from build123d import *

# Parameters (mm, degrees)
SKETCH1_W                  = 109.5
SKETCH1_H                  = 83
BOSS_EXTRUDE1_DEPTH        = 2
F_3_2_3_2_DIAMETER_HOLE2_D = 3.2
F_2_6_2_6_DIAMETER_HOLE2_D = 2.6
F_2_6_2_6_DIAMETER_HOLE1_D = 2.6
SKETCH9_R                  = 3
CUT_EXTRUDE1_DEPTH         = 1
F_2_2_2_2_DIAMETER_HOLE1_D = 2.2
FILLET1_R                  = 1
FILLET2_R                  = 3


with BuildPart() as part:
    # Sketch1 → Boss-Extrude1 (new body)
    with BuildSketch(Plane.XY):
        with Locations((0, -41.5)):
            Rectangle(SKETCH1_W, SKETCH1_H)
        with BuildLine():
            Line((-44.75, -31.5), (-48.75, -31.5))
            Line((-48.75, -31.5), (-48.75, -51.5))
            Line((-48.75, -51.5), (-44.75, -51.5))
            Line((-44.75, -51.5), (-44.75, -74))
            ThreePointArc((-44.75, -74), (-43.871320344, -76.121320344), (-41.75, -77))
            Line((-41.75, -77), (41.75, -77))
            ThreePointArc((41.75, -77), (43.871320344, -76.121320344), (44.75, -74))
            Line((44.75, -74), (44.75, -51.5))
            Line((44.75, -51.5), (48.75, -51.5))
            Line((48.75, -51.5), (48.75, -41.5))
            Line((48.75, -41.5), (48.75, -31.5))
            Line((48.75, -31.5), (44.75, -31.5))
            Line((44.75, -31.5), (44.75, -19.1))
            ThreePointArc((44.75, -19.1), (43.871320344, -16.978679656), (41.75, -16.1))
            Line((41.75, -16.1), (31.75, -16.1))
            ThreePointArc((31.75, -16.1), (29.628679656, -15.221320344), (28.75, -13.1))
            Line((28.75, -13.1), (28.75, -9))
            ThreePointArc((28.75, -9), (27.871320344, -6.878679656), (25.75, -6))
            Line((25.75, -6), (-41.75, -6))
            ThreePointArc((-41.75, -6), (-43.871320344, -6.878679656), (-44.75, -9))
            Line((-44.75, -9), (-44.75, -31.5))
        make_face(mode=Mode.SUBTRACT)
    extrude(amount=BOSS_EXTRUDE1_DEPTH)

    # Ø3.2 (3.2) Diameter Hole2 (through all)
    with Locations(Plane.XY.offset(2)):
        with Locations((-48.25, -3.5), (-48.25, -79.5), (48.25, -79.5), (48.25, -3.5)):
            Hole(F_3_2_3_2_DIAMETER_HOLE2_D / 2)

    # Ø2.6 (2.6) Diameter Hole2 (through all)
    with Locations(Plane.XY.offset(2)):
        with Locations((33.65, -11.6)):
            Hole(F_2_6_2_6_DIAMETER_HOLE2_D / 2)

    # Ø2.6 (2.6) Diameter Hole1 (through all)
    with Locations(Plane.XY.offset(2)):
        with Locations((33.65, -2.07)):
            Hole(F_2_6_2_6_DIAMETER_HOLE1_D / 2)

    # Sketch9 → Cut-Extrude1 (cut)
    with BuildSketch(Plane.XY.offset(2)):
        with Locations((-48.25, -3.5)):
            Circle(SKETCH9_R)
        with Locations((48.25, -3.5)):
            Circle(SKETCH9_R)
        with Locations((48.25, -79.5)):
            Circle(SKETCH9_R)
        with Locations((-48.25, -79.5)):
            Circle(SKETCH9_R)
    extrude(amount=-CUT_EXTRUDE1_DEPTH, mode=Mode.SUBTRACT)

    # Ø2.2 (2.2) Diameter Hole1 (through all)
    with Locations(Plane.XY.offset(2)):
        with Locations((-24.75, -3), (24.75, -3), (-24.75, -80), (24.75, -80)):
            Hole(F_2_2_2_2_DIAMETER_HOLE1_D / 2)

    # Fillet1
    fillet1_edges = [part.edges().sort_by_distance(p)[0] for p in [
        (-44.75, -31.5, 1),
        (-44.75, -51.5, 1),
        (44.75, -51.5, 1),
        (44.75, -31.5, 1),
    ]]
    fillet(fillet1_edges, radius=FILLET1_R)

    # Fillet2
    fillet2_edges = [part.edges().sort_by_distance(p)[0] for p in [
        (48.75, -31.5, 1),
        (48.75, -51.5, 1),
        (-48.75, -51.5, 1),
        (-48.75, -31.5, 1),
    ]]
    fillet(fillet2_edges, radius=FILLET2_R - 0.0001)  # a hair under: the kernel refuses the full size


solid = part.part
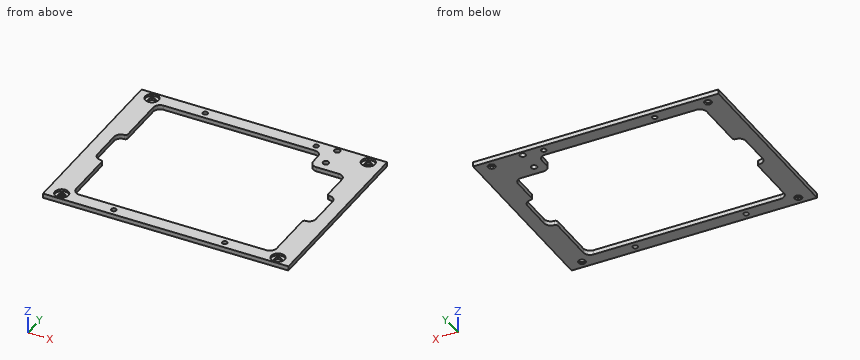
Check sheet for the modelled part. Datum: model origin and axes. Units: mm. Round coordinates to 2 decimals unless told otherwise and drop trailing zeros. Loops run counter-clockwise (first coordinate to the right, second up) from the corner with the lowest first, then second, coordinate; pieces in that order, holes last. Notation, with made-up numbers: (49, 87) - (56, 87) arc R18 ccw to (56, 98) - close; hole circle Ø10 at (9, 18.5). An arc over 180 degrees is marked (long way). Answer as CSV lines item,"result". Start each with the question number.
Item 1: Section check D-D (y = -71). Record the boundary of the cut face in (x, z).
Item 2: Section check A-A (x = 8.5). Record the boundary of the cut face in (y, z), and give its area (3 significant figures).
Item 3: Scan lines: line 1 (Y direction, x = -21.5, z = 0.9); line 2 (Y direction, x = -49.5, z = 0.65); line 3 (X direction, y = -57.5, z = 0.7). Record each from-to range of solid material in increasing order. Write a range as [from, to].
Item 4: Section check C-C (x = -24.75). Record the boundary of the cut face in (y, z).
Item 5: Section check B-B (y = -11.6). Record the boundary of the cut face in (x, z).
Item 6: Depth check by flat-ended pin: P1, Ø6.5, axis at x = 48, y = -81, coming from the +Z side; P2, Ø2, axis at x = -24.75, y = -80, coming from the +Z side; P3, Ø5, axis at x = 48.25, y = -79.5, coming from the +Z side. Enter the tip coordinate at first touch or a pass-through.
Report:
1,outline,"(-54.75, 0) - (-44.75, 0) - (-44.75, 2) - (-54.75, 2) - close; (44.75, 0) - (54.75, 0) - (54.75, 2) - (44.75, 2) - close"
2,outline,"(-83, 0) - (-77, 0) - (-77, 2) - (-83, 2) - close; (-6, 0) - (0, 0) - (0, 2) - (-6, 2) - close"
2,area,"24.0 mm2"
3,line 1,"y = [-83, -77], [-6, 0]"
3,line 2,"y = [-83, -80.5], [-78.5, -4.5], [-2.5, 0]"
3,line 3,"x = [-54.75, -44.75], [44.75, 54.75]"
4,outline,"(-83, 0) - (-81.1, 0) - (-81.1, 2) - (-83, 2) - close; (-78.9, 0) - (-77, 0) - (-77, 2) - (-78.9, 2) - close; (-6, 0) - (-4.1, 0) - (-4.1, 2) - (-6, 2) - close; (-1.9, 0) - (0, 0) - (0, 2) - (-1.9, 2) - close"
5,outline,"(-54.75, 0) - (-44.75, 0) - (-44.75, 2) - (-54.75, 2) - close; (28.75, 0) - (32.35, 0) - (32.35, 2) - (28.75, 2) - close; (34.95, 0) - (54.75, 0) - (54.75, 2) - (34.95, 2) - close"
6,P1,"stops at z = 2"
6,P2,"passes through"
6,P3,"stops at z = 1"
